```python
from build123d import *

# Parameters (mm, degrees)
SKETCH_1_R      = 7.905
SKETCH_1_R_2    = 1.75
SKETCH_1_R_3    = 1.65
SKETCH_1_W      = 40.5
SKETCH_1_H      = 20.2
EXTRUDE_1_DEPTH = 5


with BuildPart() as part:
    # 草图1 → 凸台-拉伸1 (new body)
    with BuildSketch(Plane.XY):
        with BuildLine():
            Line((106.5, -30), (-106.5, -30))
            ThreePointArc((-106.5, -30), (-110.035533906, -28.535533906), (-111.5, -25))
            Line((-111.5, -25), (-111.5, 25))
            ThreePointArc((-111.5, 25), (-110.035533906, 28.535533906), (-106.5, 30))
            Line((-106.5, 30), (106.5, 30))
            ThreePointArc((106.5, 30), (110.035533906, 28.535533906), (111.5, 25))
            Line((111.5, 25), (111.5, -25))
            ThreePointArc((111.5, -25), (110.035533906, -28.535533906), (106.5, -30))
        make_face()
        with Locations((-80, 0)):
            Circle(SKETCH_1_R, mode=Mode.SUBTRACT)
        with Locations((80, 0)):
            Circle(SKETCH_1_R, mode=Mode.SUBTRACT)
        with Locations((33.788860906, -4.762314657)):
            Circle(SKETCH_1_R_2, mode=Mode.SUBTRACT)
        with Locations((33.788860906, 5.237685343)):
            Circle(SKETCH_1_R_2, mode=Mode.SUBTRACT)
        with Locations((-14.211139094, -4.762314657)):
            Circle(SKETCH_1_R_2, mode=Mode.SUBTRACT)
        with Locations((-14.211139094, 5.237685343)):
            Circle(SKETCH_1_R_2, mode=Mode.SUBTRACT)
        with Locations((-94.849242405, 14.849242405)):
            Circle(SKETCH_1_R_2, mode=Mode.SUBTRACT)
        with Locations((-94.849242405, -14.849242405)):
            Circle(SKETCH_1_R_2, mode=Mode.SUBTRACT)
        with Locations((-65.150757595, 14.849242405)):
            Circle(SKETCH_1_R_2, mode=Mode.SUBTRACT)
        with Locations((-65.150757595, -14.849242405)):
            Circle(SKETCH_1_R_2, mode=Mode.SUBTRACT)
        with Locations((65.150757595, -14.849242405)):
            Circle(SKETCH_1_R_2, mode=Mode.SUBTRACT)
        with Locations((94.849242405, -14.849242405)):
            Circle(SKETCH_1_R_2, mode=Mode.SUBTRACT)
        with Locations((65.150757595, 14.849242405)):
            Circle(SKETCH_1_R_2, mode=Mode.SUBTRACT)
        with Locations((94.849242405, 14.849242405)):
            Circle(SKETCH_1_R_2, mode=Mode.SUBTRACT)
        with Locations((-89.5, 9.5)):
            Circle(SKETCH_1_R_2, mode=Mode.SUBTRACT)
        with Locations((-89.5, -9.5)):
            Circle(SKETCH_1_R_2, mode=Mode.SUBTRACT)
        with Locations((-70.5, 9.5)):
            Circle(SKETCH_1_R_2, mode=Mode.SUBTRACT)
        with Locations((-70.5, -9.5)):
            Circle(SKETCH_1_R_2, mode=Mode.SUBTRACT)
        with Locations((89.5, -9.5)):
            Circle(SKETCH_1_R_2, mode=Mode.SUBTRACT)
        with Locations((62, -8.868327509)):
            Circle(SKETCH_1_R_3, mode=Mode.SUBTRACT)
        with Locations((70.5, 9.5)):
            Circle(SKETCH_1_R_2, mode=Mode.SUBTRACT)
        with Locations((89.5, 9.5)):
            Circle(SKETCH_1_R_2, mode=Mode.SUBTRACT)
        with Locations((9.788860906, 0.237685343)):
            Rectangle(SKETCH_1_W, SKETCH_1_H, mode=Mode.SUBTRACT)
    extrude(amount=EXTRUDE_1_DEPTH)


solid = part.part
```
Could you check a few things on this model? Use its own coordinates, in mm. A direction names the side the tool comes from. Give positions to 0.01 mm unless a question says otherwise; leave off trailing zeros. Write each loop counter-clockwise with the first axis right and the second up, starting at its lowest first coordinate (ties: lowest second). Pieces come first, ordered by that corner, then holes. Notation, with made-up numbers: (45.5, 63) - (102.5, 63) arc R16 cw to (102.5, 84) - close; hole circle Ø11 at (10.25, 72.25). An arc over 180 degrees is marked (long way). One line per item, written item: value. Start each with the question number.
Item 1: Which directions (+Z, -Z, +X, -X, +Y, -Y) give clear straight access to the entire face, cutting with the end or side of a thin tool? Please do faces 4 (the face through (10, -9.862, 2)), 5 (the face through (1, -30, 2)).
Item 2: If we mould it in two halves opening along X, with no side actions, what happens to faces 1 (the face through (2, 14, 0)), 2 (the face through (111.5, 0, 2)), 3 (the face through (-72.46, 2.37, 2.46))? For each: +X half, -X half, draft (parallel to the pull), parting line (faces both ways), or undercut.
Item 3: Please list where these lines run through material, in increasing order: line 1 (X direction, y = -15, z = 1.2); line 2 (Y direction, x = -70.5, z = 1.75); line 3 (Y direction, x = 62, z = 1.45). Write a range as from..to.
Item 4: Imagine slicing it at B-B, the plane y = 0. List the corners of the cut face in (x, z) for me (3 decimals), and give its area (3 significant figures).
Item 5: Imagine slicing it at A-A, the plane x = 80. List the corners of the cut face in (y, z) for me (3 decimals), and give its area (3 significant figures).
Item 6: Imagine slicing it at C-C, the plane z = 1.95. Give the number of separate pieces and of enclosed holes in the cut face, and give its area (3 significant figures).
Item 7: I'm going to push a flat-ended pin straight in: pin 1 (2 mm diameter, centred on x = 85, y = 16.5, fed in from -Z). Where does the tip first touch, or does it pass through?
Geometry says:
1. face 4: +Z, -Z
1. face 5: +Z, -Z, +X, -X, -Y
2. face 1: draft
2. face 2: +X half
2. face 3: undercut
3. line 1: -111.5..-96.59, -93.11..-66.89, -63.41..63.41, 66.89..93.11, 96.59..111.5
3. line 2: -30..-11.25, -7.75..7.75, 11.25..30
3. line 3: -30..-10.52, -7.22..30
4. outline: (-111.5, 0) - (-87.905, 0) - (-87.905, 5) - (-111.5, 5) - close; (-72.095, 0) - (-10.461, 0) - (-10.461, 5) - (-72.095, 5) - close; (30.039, 0) - (72.095, 0) - (72.095, 5) - (30.039, 5) - close; (87.905, 0) - (111.5, 0) - (111.5, 5) - (87.905, 5) - close
4. area: 754 mm^2
5. outline: (-30, 0) - (-7.905, 0) - (-7.905, 5) - (-30, 5) - close; (7.905, 0) - (30, 0) - (30, 5) - (7.905, 5) - close
5. area: 221 mm^2
6. separate pieces: 1
6. enclosed holes: 23
6. area: 12,000 mm^2
7. pin 1: z = 0
